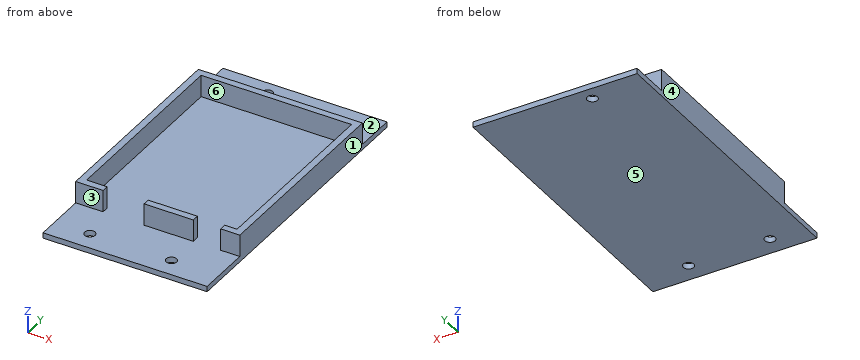
```python
from build123d import *

# Parameters (mm, degrees)
F0_W     = 60
F0_H     = 75
F1_DEPTH = 10
F2_W     = 55
F2_H     = 70
F3_DEPTH = 8
F4_W     = 15
F4_H     = 3.129633
F4_W_2   = 10
F5_DEPTH = 8
F6_W     = 60
F6_H     = 20
F6_R     = 1.905
F7_DEPTH = 2
F8_W     = 60
F8_H     = 15
F8_R     = 1.905
F9_DEPTH = 2


with BuildPart() as f1:
    # F0 (on Top) → F1 (new body)
    with BuildSketch(Plane.XY):
        with Locations((-1.779088, 0.283666)):
            Rectangle(F0_W, F0_H)
    extrude(amount=F1_DEPTH)

    # F2 (on face) → F3 (cut)
    with BuildSketch(Plane.XY.offset(10)):
        with Locations((-1.779088, 0.283666)):
            Rectangle(F2_W, F2_H)
    extrude(amount=-F3_DEPTH, mode=Mode.SUBTRACT)

    # F4 (on face) → F5 (cut)
    with BuildSketch(Plane.XY.offset(2)):
        with Locations((-14.279088, -36.044677)):
            Rectangle(F4_W, F4_H)
        with Locations((16.220912, -36.044677)):
            Rectangle(F4_W_2, F4_H)
    extrude(amount=F5_DEPTH, mode=Mode.SUBTRACT)

    # F6 (on Top) → F7 (join)
    with BuildSketch(Plane.XY):
        with Locations((-1.779088, -47.216334)):
            Rectangle(F6_W, F6_H)
        with Locations((-18.874088, -50.121334)):
            Circle(F6_R, mode=Mode.SUBTRACT)
        with Locations((10.935912, -50.121334)):
            Circle(F6_R, mode=Mode.SUBTRACT)
    extrude(amount=F7_DEPTH)

    # F8 (on Top) → F9 (join)
    with BuildSketch(Plane.XY):
        with Locations((-1.779088, 45.283666)):
            Rectangle(F8_W, F8_H)
        with Locations((-12.374088, 47.688666)):
            Circle(F8_R, mode=Mode.SUBTRACT)
    extrude(amount=F9_DEPTH)


solid = f1.part
```
Source: CAD feature listing. Evaluate the final solid. Frame: model axes, mm. Face numbers are marked on the shaded views. A direction names the side the tool comes from. Give positions to 0.01 mm unless a question says otherwise; leave off trailing zeros. Loops run counter-clockwise (first coordinate to the right, second up) from the corner with the lowest first, then second, coordinate; pieces in that order, holes last. Notation, with made-up numbers: (14, 36) -> (55, 36) arc R25 cw to (55, 53) -> close; hole circle Ø10 at (-19, 61). An arc over 180 degrees is marked (long way). Use a Markdown table: item, result. Add a question column.
(1) Section query D-D (x = 14.5). Output: boundary loops of the cut face in (y, z), then the cut area to 3 significant figures.
(2) First-contact query: pin 1 Ø2 at (x, z) = (22.5, 7) entering from +Y; pin 2 Ø2.5 at (x, y) = (-18.87, -50.12) entering from -Z; pin 3 Ø18 at (x, y) = (-6, 1) entering from +Z; pin 4 Ø6 at (x, z) = (10, 6.5) entering from -Y. Flat tips, straight axial feed; report the tip coordinate or a pass-through.
(3) Access query for the marked faces 1, 2 and 3. Directions: +Z, -Z, +X, -X, +Y, -Y. A direction counts if a zero-diameter tool reaches every point of the face in a straight line with its end or side. Return the directions, or none.
(4) Section query B-B (x = -11.5). Output: boundary loops of the cut face in (y, z), then the cut area to 3 significant figures.
(5) Section query A-A (z = 4). Output: boundary loops of the cut face in (x, y).
(6) Section query C-C (y = 2.5). Output: boundary loops of the cut face in (x, z).
(7) Pull-direction query (X, two-part tool) for the marked faces 4, 5 and 6; classes: +X half, -X half, draft (parallel to the pull), parting line (faces both ways), or undercut.
(8) Ray query, line 1 (Y direction, x = 21.5, z = 9.75); line 2 (X direction, y = -19, z = 7.75); line 3 (Z direction, x = 6.5, y = -18). Return the intervals inside material, ascending.
Checked values:
| question | item | result |
|---|---|---|
| 1 | outline | (-57.22, 0) -> (52.78, 0) -> (52.78, 2) -> (37.78, 2) -> (37.78, 10) -> (35.28, 10) -> (35.28, 2) -> (-57.22, 2) -> close |
| 1 | area | 240 mm^2 |
| 2 | pin 1 | y = 37.78 |
| 2 | pin 2 | through |
| 2 | pin 3 | z = 2 |
| 2 | pin 4 | y = -37.22 |
| 3 | face 1 | +Z, -Z, +X, +Y, -Y |
| 3 | face 2 | +Z, +X, -X, +Y |
| 3 | face 3 | +Z, +X, -X, -Y |
| 4 | outline | (-57.22, 0) -> (46, 0) -> (46, 2) -> (37.78, 2) -> (37.78, 10) -> (35.28, 10) -> (35.28, 2) -> (-57.22, 2) -> close; (49.38, 0) -> (52.78, 0) -> (52.78, 2) -> (49.38, 2) -> close |
| 4 | area | 233 mm^2 |
| 5 | outline | (-31.78, -37.22) -> (-21.78, -37.22) -> (-21.78, -34.72) -> (-29.28, -34.72) -> (-29.28, 35.28) -> (25.72, 35.28) -> (25.72, -34.72) -> (21.22, -34.72) -> (21.22, -37.22) -> (28.22, -37.22) -> (28.22, 37.78) -> (-31.78, 37.78) -> close; (-6.78, -37.22) -> (11.22, -37.22) -> (11.22, -34.72) -> (-6.78, -34.72) -> close |
| 6 | outline | (-31.78, 0) -> (28.22, 0) -> (28.22, 10) -> (25.72, 10) -> (25.72, 2) -> (-29.28, 2) -> (-29.28, 10) -> (-31.78, 10) -> close |
| 7 | face 4 | -X half |
| 7 | face 5 | draft |
| 7 | face 6 | undercut |
| 8 | line 1 | -37.22 to -34.72, 35.28 to 37.78 |
| 8 | line 2 | -31.78 to -29.28, 25.72 to 28.22 |
| 8 | line 3 | 0 to 2 |
